from build123d import *

# Parameters (mm, degrees)
SKETCH1_R           = 15
SKETCH1_R_2         = 12.5
BOSS_EXTRUDE1_DEPTH = 115
SKETCH2_W           = 8
SKETCH2_H           = 5
BOSS_EXTRUDE2_DEPTH = 115


with BuildPart() as part:
    # Sketch1 → Boss-Extrude1 (new body)
    with BuildSketch(Plane.XY):
        Circle(SKETCH1_R)
        Circle(SKETCH1_R_2, mode=Mode.SUBTRACT)
    extrude(amount=BOSS_EXTRUDE1_DEPTH)

    # Sketch2 → Boss-Extrude2 (add)
    with BuildSketch(Plane.XY):
        with Locations((0, 15)):
            Rectangle(SKETCH2_W, SKETCH2_H)
    extrude(amount=BOSS_EXTRUDE2_DEPTH)


solid = part.part
Input: part model. Units: mm. Frame: model coordinates. A direction names the side the tool comes from. Coordinates: 2 decimals unless noted, no trailing zeros. Order: outer loops, then holes, each group sorted by start corner. A loop starts at its lowest first (then second) coordinate and runs counter-clockwise, first axis right, second up.
1. Cut plane C-C, the plane z = 63.5. Return loops of the section in (x, y), plus the area to 3 significant figures.
Checked values:
outline: (-4, 14.46) arc R15 ccw (long way) to (4, 14.46) - (4, 17.5) - (-4, 17.5) - close; hole circle Ø25 at (0, 0)
area: 237 mm2
2. Cut plane B-B, the plane y = 0. Return loops of the section in (x, z), plus the area to 3 significant figures.
Checked values:
outline: (-15, 0) - (-12.5, 0) - (-12.5, 115) - (-15, 115) - close; (12.5, 0) - (15, 0) - (15, 115) - (12.5, 115) - close
area: 575 mm2
3. Cut plane A-A, the plane x = 0. Return loops of the section in (y, z), plus the area to 4 significant figures.
Checked values:
outline: (-15, 0) - (-12.5, 0) - (-12.5, 115) - (-15, 115) - close; (12.5, 0) - (17.5, 0) - (17.5, 115) - (12.5, 115) - close
area: 862.5 mm2
4. Draft query along Y for faces 3 (the cylindrical face through (11.923, 3.755, 56.695)), 4 (the flat face through (0, 17.5, 57)), 5 (the flat face through (-4, 16, 57)). Return one class per face: +Y half, -Y half, draft (parallel to the pull), parting line (faces both ways), or undercut.
Checked values:
face 3: undercut
face 4: +Y half
face 5: draft
5. Contact query for flat-ended pins moving along their axis: P1, Ø1.5, axis at y = 16, z = 44, coming from the +X side; P2, Ø3.5, axis at y = 16.5, z = 56.5, coming from the -X side; P3, Ø1, axis at y = 10, z = 18.5, coming from the -X side. Output: stop coordinate, or through.
Checked values:
P1: stops at x = 4
P2: stops at x = -4
P3: stops at x = -11.61
6. Ray query, line 1 along Y through (x, z) = (0, 26); line 2 along Y through (x, z) = (11.5, 110); line 3 along X through (y, z) = (15.5, 23). Return the intervals inside material, ascending.
Checked values:
line 1: y = -15 to -12.5, 12.5 to 17.5
line 2: y = -9.63 to -4.9, 4.9 to 9.63
line 3: x = -4 to 4
7. Access query for faces 1 (the cylindrical face through (-0.603, -14.988, 56.695)), 2 (the flat face through (4, 16, 57)). Directions: +Z, -Z, +X, -X, +Y, -Y. A direction counts if a zero-diameter tool reaches every point of the face in a straight line with its end or side. Return the directions, or none.
Checked values:
face 1: +Z, -Z
face 2: +Z, -Z, +X, +Y
